Geometry check sheet. Reference: the model listing, model coordinates, mm. A direction names the side the tool comes from. Round coordinates to 2 decimals unless told otherwise and drop trailing zeros. Order: outer loops, then holes, each group sorted by start corner. A loop starts at its lowest first (then second) coordinate and runs counter-clockwise, first axis right, second up. Notation, with made-up numbers: (-0.5, -38) -> (5.5, -38) arc R23 ccw to (5.5, 0) -> close; hole circle Ø2 at (-6, 78). An arc over 180 degrees is marked (long way). Use a Markdown table: item, result. Add a question column.
Item 1: Gauge pin test, flat ends, axial feed: pin 1 Ø10 at (x, z) = (10, -44) entering from +Y; pin 2 Ø5 at (x, z) = (3, -36.5) entering from -Y; pin 3 Ø8 at (x, z) = (0, -20.5) entering from -Y. Record the tip position at first contact, or that the pin passes through.
Item 2: Material ranges on probe 1 along Y at (x, z) = (-3.25, -27); probe 2 along Y at (x, z) = (10.25, -53); probe 3 along X at (y, z) = (-6.75, -48), recorded low to high. Write a range as [from, to].
Item 3: Mould release check, pull along Z, two halves, no side actions. Record for faces 4 (the flat face through (11, -7, -34)), 5 (the flat face through (-5, 10, -12)), 6 (the flat face through (3, -11, -10)), 7 (the flat face through (2.5, 10, -5)): pulls with the +Z half, pulls with the -Z half, needs draft (parallel to the pull), parting line crosses it, or undercut.
Item 4: Sectioned sample at B-B, the plane z = -21. Record the cut outline in (x, y).
Item 5: Set-up check for faces 1 (the flat face through (0, 0, -56)), 2 (the cylindrical face through (0, 10, -12)), 3 (the cylindrical face through (0, -12, -6)): record each of +Z, -Z, +X, -X, +Y, -Y from which the full face is reachable in a straight line by a thin tool's end or side.
Item 6: Sectioned sample at A-A, the plane z = -49.5. Record the cut outline in (x, y), and give its area (3 significant figures).
from build123d import *

# Parameters (mm, degrees)
CUT_EXTRUDE_1_DEPTH = 63.745517768
CHAMFER_1_SIZE      = 1
CHAMFER_2_SIZE      = 0.5


with BuildPart() as part:
    # 草图1 → 旋转1 (revolve)
    with BuildSketch(Plane(origin=(0, 0, 0), x_dir=(0, 0, -1), z_dir=(1, 0, 0)), mode=Mode.PRIVATE) as revolve_1_sk:
        Polygon((0, 0), (0, 12), (10, 12), (10, 11), (12, 11), (12, 12.5), (34, 12.5), (34, 15), (56, 15), (56, 0), align=None)
    revolve(revolve_1_sk.sketch.rotate(Axis((0, 0, 0), (0, 0, -1)), 90), axis=Axis((0, 0, 0), (0, 0, -1)))

    # 草图2 → 切除-拉伸1 (cut, through all)
    with BuildSketch(Plane(origin=(0, 9, 0), x_dir=(1, 0, 0), z_dir=(0, 1, 0))):
        with BuildLine():
            Line((-2.5, 9.5), (-2.5, 0))
            Line((-2.5, 0), (2.5, 0))
            Line((2.5, 0), (2.5, 9.5))
            ThreePointArc((2.5, 9.5), (0, 12), (-2.5, 9.5))
        make_face()
    extrude(amount=CUT_EXTRUDE_1_DEPTH, mode=Mode.SUBTRACT)

    # 倒角1
    chamfer_1_edges = [part.edges().sort_by_distance(p)[0] for p in [
        (0, -12, 0),
    ]]
    chamfer(chamfer_1_edges, length=CHAMFER_1_SIZE)

    # 倒角2
    # the kernel refuses this chamfer: 0.5 mm, written as the material it takes off along each edge
    with BuildSketch(Plane(origin=(0, 0, -34), x_dir=(1, 0, 0), z_dir=(0, 1, 0))) as chamfer_2_piece_1:
        Polygon((15 - CHAMFER_2_SIZE, 0), (15, CHAMFER_2_SIZE), (15, 0), align=None)
    revolve(axis=Axis((0, 0, -34), (0, 0, -1)), mode=Mode.SUBTRACT)
    with BuildSketch(Plane(origin=(0, 0, -12), x_dir=(0, 1, 0), z_dir=(-1, 0, 0))) as chamfer_2_piece_2:
        Polygon((12.5 - CHAMFER_2_SIZE, 0), (12.5, CHAMFER_2_SIZE), (12.5, 0), align=None)
    revolve(axis=Axis((0, 0, -12), (0, 0, -1)), revolution_arc=90, mode=Mode.SUBTRACT)
    with BuildSketch(Plane(origin=(0, 0, -12), x_dir=(1, 0, 0), z_dir=(0, 1, 0))) as chamfer_2_piece_3:
        Polygon((12.5 - CHAMFER_2_SIZE, 0), (12.5, CHAMFER_2_SIZE), (12.5, 0), align=None)
    revolve(axis=Axis((0, 0, -12), (0, 0, -1)), revolution_arc=270, mode=Mode.SUBTRACT)


solid = part.part
Found:
| question | item | result |
|---|---|---|
| 1 | pin 1 | stops at y = 14.14 |
| 1 | pin 2 | stops at y = -14.99 |
| 1 | pin 3 | stops at y = -12.5 |
| 2 | probe 1 | y = [-12.07, 12.07] |
| 2 | probe 2 | y = [-10.95, 10.95] |
| 2 | probe 3 | x = [-13.4, 13.4] |
| 3 | face 4 | pulls with the +Z half |
| 3 | face 5 | undercut |
| 3 | face 6 | undercut |
| 3 | face 7 | needs draft |
| 4 | outline | circle Ø25 at (0, 0) |
| 5 | face 1 | -Z, +X, -X, +Y, -Y |
| 5 | face 2 | +Z, +Y |
| 5 | face 3 | +Z |
| 6 | outline | circle Ø30 at (0, 0) |
| 6 | area | 707 mm2 |
